Design review of the part shown in the three views and the two pictorial views. Dimensions are in mm from the part's minimum x, y and z. Round coordinates to 2 decimals unless told otherwise and drop trailing zeros. Write each loop counter-clockwise with the first axis right and the second up, starting at its lowest first coordinate (ties: lowest second). Pieces come first, ordered by that corner, then holes. Notation, with made-up numbers: (-38.75, -19.5) -> (-14.75, -19.5) arc R30 ccw to (-14.75, 3.5) -> close; hole circle Ø1 at (41, 45.5). An arc over 180 degrees is marked (long way). Answer as a JSON object with one key per item and string values. Group by question number.
1) Insertion check: pin 1 Ø1.5 at (x, y) = (16.5, 16) entering from -Z (1 decimal); pin 2 Ø2.5 at (x, y) = (7.24, 4.81) entering from +Z; pin 3 Ø1.5 at (y, z) = (12, 9) entering from -X; pin 4 Ø4 at (x, z) = (2.5, 9.5) entering from -Y. Each pin has a flat end and moves straight along its axis. Give the tip position at first contact, or say it passes through.
2) To check wall thickness, follow probe 1 along X at (y, z) = (3.75, 16.5) (1 decimal); probe 2 along Y at (x, z) = (12.75, 16.75) (1 decimal); probe 3 along Y at (x, z) = (9.75, 27.5) (1 decimal). State the ranges of each line that lie inside material, in increasing order. Write a range as [from, to].
3) We need section A-A, the plane z = 12. Write out the cut boundary in (x, y) (1 decimal), then the cut area to 3 significant figures.
4) We need section C-C, the plane x = 9.5. Write out the cut boundary in (y, z), then the cut area to 3 significant figures.
5) Mouldability with a two-part tool opening along Y and no side actions: class the marked faces 1, 2 and 3 as pulls with the +Y half, pulls with the -Y half, needs draft (parallel to the pull), parting line crosses it, or undercut.
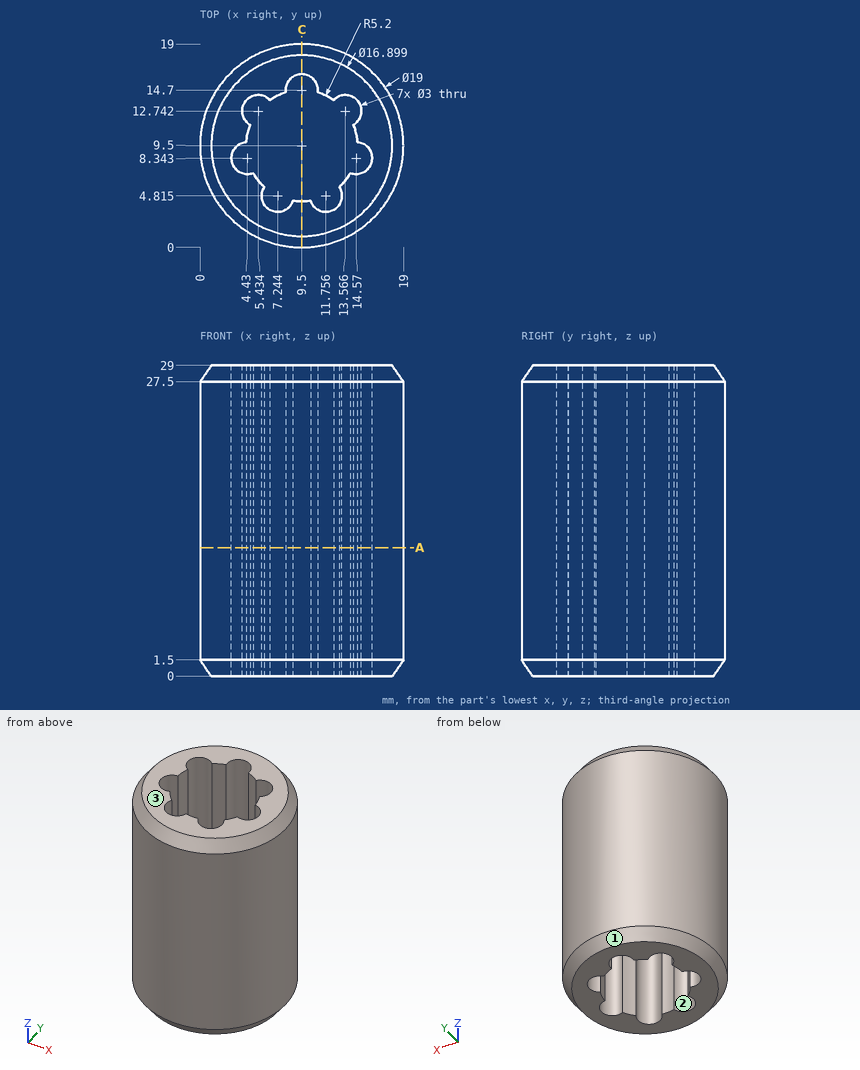
Here are the results:
{
 "1": {"pin 1": "stops at z = 0.5", "pin 2": "passes through", "pin 3": "stops at x = 0.16", "pin 4": "stops at y = 1.42"},
 "2": {"probe 1": "x = [1.9, 6.2], [8.3, 10.7], [12.8, 17.1]", "probe 2": "y = [0.6, 3.7], [14, 18.4]", "probe 3": "y = [0, 4.3], [16.2, 19]"},
 "3": {"outline": "circle Ø19 at (9.5, 9.5); hole (4.3, 9.8) arc R1.5 ccw (long way) to (5, 6.9) arc R5.2 ccw to (6, 5.7) arc R1.5 ccw (long way) to (8.7, 4.4) arc R5.2 ccw to (10.3, 4.4) arc R1.5 ccw (long way) to (13, 5.7) arc R5.2 ccw to (14, 6.9) arc R1.5 ccw (long way) to (14.7, 9.8) arc R5.2 ccw to (14.3, 11.4) arc R1.5 ccw (long way) to (12.5, 13.8) arc R5.2 ccw to (11, 14.5) arc R1.5 ccw (long way) to (8, 14.5) arc R5.2 ccw to (6.5, 13.8) arc R1.5 ccw (long way) to (4.7, 11.4) arc R5.2 ccw to start", "area": "172 mm^2"},
 "4": {"outline": "(0, 1.5) -> (1.05, 0) -> (4.3, 0) -> (4.3, 29) -> (1.05, 29) -> (0, 27.5) -> close; (16.2, 0) -> (17.95, 0) -> (19, 1.5) -> (19, 27.5) -> (17.95, 29) -> (16.2, 29) -> close", "area": "203 mm^2"},
 "5": {"face 1": "parting line crosses it", "face 2": "undercut", "face 3": "needs draft"}
}
